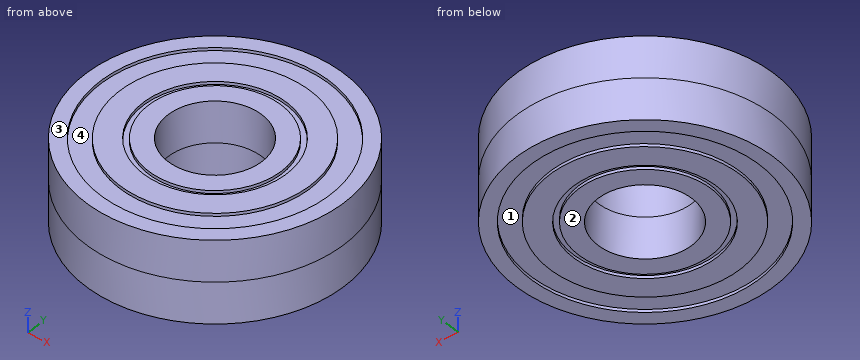
from build123d import *

# Parameters (mm, degrees)
F0_R     = 11
F0_R_2   = 9.75
F0_R_3   = 8.1
F0_R_4   = 6.1
F0_R_5   = 5.65
F0_R_6   = 4
F1_DEPTH = 3.5
F2_DEPTH = 0.25


with BuildPart() as f1:
    # F0 (on Top) → F1 (new body)
    with BuildSketch(Plane.XY):
        Circle(F0_R)
        Circle(F0_R_2, mode=Mode.SUBTRACT)
        Circle(F0_R_2)
        Circle(F0_R_3, mode=Mode.SUBTRACT)
        Circle(F0_R_3)
        Circle(F0_R_4, mode=Mode.SUBTRACT)
        Circle(F0_R_4)
        Circle(F0_R_5, mode=Mode.SUBTRACT)
        Circle(F0_R_5)
        Circle(F0_R_6, mode=Mode.SUBTRACT)
    extrude(amount=F1_DEPTH)

    # F0 (on Top) → F2 (cut)
    with BuildSketch(Plane.XY):
        Circle(F0_R_2)
        Circle(F0_R_3, mode=Mode.SUBTRACT)
        Circle(F0_R_4)
        Circle(F0_R_5, mode=Mode.SUBTRACT)
    extrude(amount=F2_DEPTH, mode=Mode.SUBTRACT)

    # F3: F1 across face


with BuildPart() as f1_1:
    add(f1.part)
    add(f1.part.mirror(Plane.XY.offset(3.5)))


solid = f1_1.part
Could you check a few things on this model? Use its own coordinates, in mm. Face numbers are marked on the shaded views. A direction names the side the tool comes from. Round coordinates to 2 decimals unless told otherwise and drop trailing zeros. Loops run counter-clockwise (first coordinate to the right, second up) from the corner with the lowest first, then second, coordinate; pieces in that order, holes last. Notation, with made-up numbers: (62, -2.75) - (102, -2.75) arc R16 ccw to (102, 19.25) - close; hole circle Ø8 at (-8.5, -23.75). An arc over 180 degrees is marked (long way). Write item = value, one per line.
1) Imagine slicing it at B-B (y = 7). Please give me the cut outline in (x, z), and give its area (3 significant figures).
Computed:
outline = (-8.49, 0) - (-6.79, 0) - (-6.79, 0.25) - (-4.08, 0.25) - (-4.08, 0) - (4.08, 0) - (4.08, 0.25) - (6.79, 0.25) - (6.79, 0) - (8.49, 0) - (8.49, 7) - (6.79, 7) - (6.79, 6.75) - (4.08, 6.75) - (4.08, 7) - (-4.08, 7) - (-4.08, 6.75) - (-6.79, 6.75) - (-6.79, 7) - (-8.49, 7) - close
area = 116 mm2
2) Imagine slicing it at D-D (y = -9). Please give me the cut outline in (x, z), and give its area (3 significant figures).
Computed:
outline = (-6.32, 0) - (-3.75, 0) - (-3.75, 0.25) - (3.75, 0.25) - (3.75, 0) - (6.32, 0) - (6.32, 7) - (3.75, 7) - (3.75, 6.75) - (-3.75, 6.75) - (-3.75, 7) - (-6.32, 7) - close
area = 84.8 mm2
3) I'm going to push flat-ended pins straight in: P1, Ø2, axis at x = -7, z = 1.5, coming from the +Y side; P2, Ø3, axis at y = 6, z = 1.5, coming from the +X side; P3, Ø6.5, axis at x = 0, y = 0, coming from the -Z side; P4, Ø1.5, axis at y = 3, z = 6, coming from the +X side. Where does each tip first touch, or does it pass through?
Computed:
P1 = 9.22
P2 = 10.04
P3 = through
P4 = 10.77
4) If we mould it in two halves opening along X, with no side actions, what happens to the marked faces 1 and 2? For each: pulls with the +X half, pulls with the -X half, needs draft (parallel to the pull), parting line crosses it, or undercut.
Computed:
face_1 = undercut
face_2 = needs draft
5) I need wall thicknesses on line 1 along Y through (x, z) = (0, 6.85); line 2 along Y through (x, z) = (0, 2.05); line 3 along X through (y, z) = (2.25, 6). Which ranges of each line are inside material? Lowest first, please. Write a range as from..to.
Computed:
line_1 = -11..-9.75, -8.1..-6.1, -5.65..-4, 4..5.65, 6.1..8.1, 9.75..11
line_2 = -11..-4, 4..11
line_3 = -10.77..-3.31, 3.31..10.77
6) On a 3-axis mill with a long thin cutter (end or side, diameter ignored), from which of +Z, -Z, +X, -X, +Y, -Y can I reach the whole of each face in a straight line? I mean the marked faces 3 and 4. Say none if no direction works.
Computed:
face_3 = +Z, +X, -X, +Y, -Y
face_4 = +Z
7) Imagine slicing it at A-A (z = 4.5). Please give me the cut outline in (x, y), and give its area (3 significant figures).
Computed:
outline = circle Ø22 at (0, 0); hole circle Ø8 at (0, 0)
area = 330 mm2
